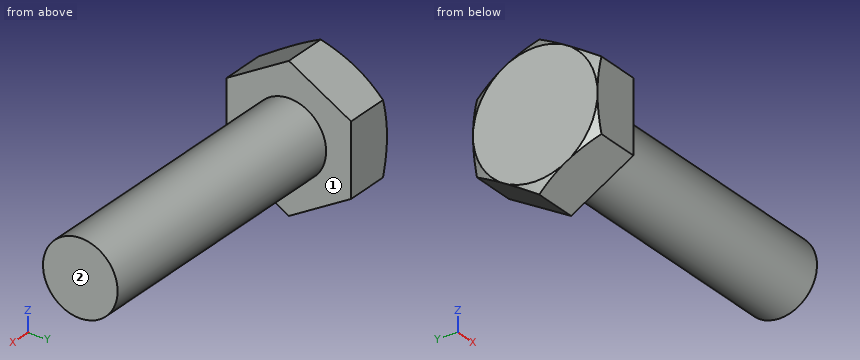
```python
from build123d import *

# Parameters (mm, degrees)
SKETCH2_R           = 3
BOSS_EXTRUDE1_DEPTH = 23.2
BOSS_EXTRUDE2_DEPTH = 4


with BuildPart() as part:
    # Sketch2 → Boss-Extrude1 (new body)
    with BuildSketch(Plane(origin=(0, 0, 0), x_dir=(0, 0, -1), z_dir=(1, 0, 0))):
        Circle(SKETCH2_R)
    extrude(amount=BOSS_EXTRUDE1_DEPTH)

    # Sketch3 → Boss-Extrude2 (add)
    with BuildSketch(Plane.ZY):
        Polygon((5.773502692, 0), (2.886751346, 5), (-2.886751346, 5), (-5.773502692, 0), (-2.886751346, -5), (2.886751346, -5), align=None)
    extrude(amount=BOSS_EXTRUDE2_DEPTH)

    # Sketch5 → Cut-Revolve1 (revolve, cut)
    with BuildSketch(Plane(origin=(0, 0, 0), x_dir=(1, 0, 0), z_dir=(0, 1, 0))):
        Polygon((-4, 5), (-4, 5.773502692), (-3.553418013, 5.773502692), align=None)
    revolve(axis=Axis((23.2, 0, 0), (-1, 0, 0)), mode=Mode.SUBTRACT)


solid = part.part
```
Here's how the part is built. I have some questions about the finished solid (model axes, mm). Face numbers are marked on the shaded views. A direction names the side the tool comes from. Coordinates: 2 decimals unless noted, no trailing zeros. Write each loop counter-clockwise with the first axis right and the second up, starting at its lowest first coordinate (ties: lowest second). Pieces come first, ordered by that corner, then holes. Notation, with made-up numbers: (-22, -15.75) - (-13, -15.75) arc R23 cw to (-13, 23.25) - close; hole circle Ø8 at (-17.5, -2). An arc over 180 degrees is marked (long way). One line per item, written item: value.
1) I need wall thicknesses on line 1 along X through (y, z) = (-3.5, 2.5); line 2 along Z through (x, y) = (7.75, -0.5); line 3 along Y through (x, z) = (-2, 4.5). Which ranges of each line are inside material? Lowest first, please.
Model answer:
line 1: x = -4 to 0
line 2: z = -2.96 to 2.96
line 3: y = -2.21 to 2.21
2) Suppose I cut it at A-A on x = 12. Write out the boundary of the cut face in (y, z).
Model answer:
outline: circle Ø6 at (0, 0)
3) I'm going to push flat-ended pins straight in: P1, Ø4, axis at x = 16.5, z = -1, coming from the -Y side; P2, Ø5, axis at x = 3.5, y = -0.5, coming from the +Z side; P3, Ø1.5, axis at x = 18.5, y = -3.5, coming from the -Z side; P4, Ø1, axis at x = 16, z = 4, coming from the -Y side. Where does each tip first touch, or does it pass through?
Model answer:
P1: stops at y = -3
P2: stops at z = 3
P3: stops at z = -1.2
P4: passes through
4) On a 3-axis mill with a long thin cutter (end or side, diameter ignored), from which of +Z, -Z, +X, -X, +Y, -Y can I reach the whole of each face in a straight line? I mean the marked faces 1 and 2. Say none if no direction works.
Model answer:
face 1: +X
face 2: +Z, -Z, +X, +Y, -Y
